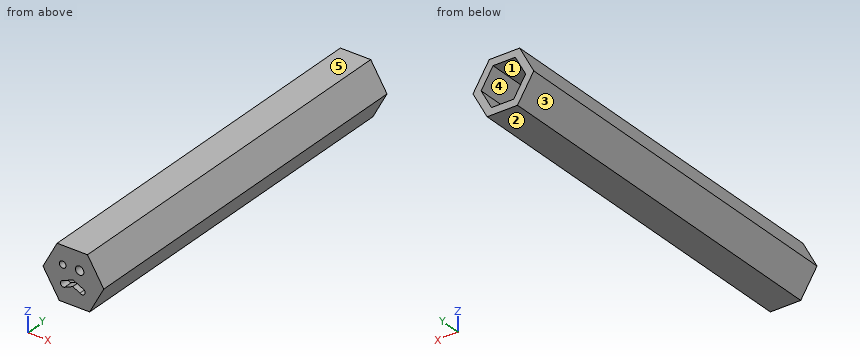
from build123d import *

# Parameters (mm, degrees)
F1_DEPTH = 31.75
F2_R     = 0.5886867957
F2_R_2   = 0.7557919615
F3_DEPTH = 1.5875


with BuildPart() as f1:
    # F0 (on Front) → F1 (new body, symmetric)
    with BuildSketch(Plane.XZ):
        Polygon((5.4726746476, 0.2241786608), (2.5421929086, 4.8515646018), (-2.930481739, 4.6273859411), (-5.4726746476, -0.2241786608), (-2.5421929086, -4.8515646018), (2.930481739, -4.6273859411), align=None)
        Polygon((-2.1458815411, 3.3884606556), (1.8615522369, 3.5526182559), (4.0074337781, 0.1641576003), (2.1458815411, -3.3884606556), (-1.8615522369, -3.5526182559), (-4.0074337781, -0.1641576003), align=None, mode=Mode.SUBTRACT)
    extrude(amount=F1_DEPTH, both=True)

    # F2 (on face) → F3 (join)
    with BuildSketch(Plane.XZ.offset(31.75)):
        Polygon((-2.5421929086, -4.8515646018), (2.930481739, -4.6273859411), (5.4726746476, 0.2241786608), (2.5421929086, 4.8515646018), (-2.930481739, 4.6273859411), (-5.4726746476, -0.2241786608), align=None)
        Polygon((-1.8615522369, -3.5526182559), (-4.0074337781, -0.1641576003), (-2.1458815411, 3.3884606556), (1.8615522369, 3.5526182559), (4.0074337781, 0.1641576003), (2.1458815411, -3.3884606556), align=None, mode=Mode.SUBTRACT)
        Polygon((-2.1458815411, 3.3884606556), (-4.0074337781, -0.1641576003), (-1.8615522369, -3.5526182559), (2.1458815411, -3.3884606556), (4.0074337781, 0.1641576003), (1.8615522369, 3.5526182559), align=None)
        with BuildLine():
            ThreePointArc((-1.6080282877, -2.2762045416), (-2.3121206431, -1.9400866098), (-1.90285574, -1.2758400079))
            Line((-1.90285574, -1.2758400079), (-0.0846300536, -0.4070492287))
            Line((-0.0846300536, -0.4070492287), (1.6315181704, -1.1626920101))
            ThreePointArc((1.6315181704, -1.1626920101), (1.7606026884, -1.201756272), (1.8765772228, -1.270594755))
            ThreePointArc((1.8765772228, -1.270594755), (1.9710769764, -2.063707268), (1.1761976946, -2.1419670217))
            Line((1.1761976946, -2.1419670217), (-0.1107579301, -1.5566768125))
            Line((-0.1107579301, -1.5566768125), (-1.5564763423, -2.2514307564))
            ThreePointArc((-1.5564763423, -2.2514307564), (-1.5819143346, -2.2645209548), (-1.6080282877, -2.2762045416))
        make_face(mode=Mode.SUBTRACT)
        with Locations((-1.9266997697, 1.430987264)):
            Circle(F2_R, mode=Mode.SUBTRACT)
        with Locations((1.1305541266, 1.6205844004)):
            Circle(F2_R_2, mode=Mode.SUBTRACT)
    extrude(amount=F3_DEPTH)


solid = f1.part
Could you check a few things on this model? Use its own coordinates, in mm. Face numbers are marked on the shaded views. A direction names the side the tool comes from. Give positions to 0.01 mm unless a question says otherwise; leave off trailing zeros. Order: outer loops, then holes, each group sorted by start corner. A loop starts at its lowest first (then second) coordinate and runs counter-clockwise, first axis right, second up.
1. Suppose I cut it at A-A (y = -17.5). Write out the boundary of the cut face in (x, z), plus the area to 3 significant figures.
Answers below:
outline: (-5.47, -0.22) - (-2.54, -4.85) - (2.93, -4.63) - (5.47, 0.22) - (2.54, 4.85) - (-2.93, 4.63) - close; hole (-4.01, -0.16) - (-1.86, -3.55) - (2.15, -3.39) - (4.01, 0.16) - (1.86, 3.55) - (-2.15, 3.39) - close
area: 36.1 mm2
2. I need wall thicknesses on L1, parallel to Y at x = -0.75, z = 0.75; L2, parallel to Z at x = -3.75, y = -24; L3, parallel to X at y = -6, z = -1. Which ranges of each line are inside material? Lowest first, please.
Answers below:
L1: y = -33.34 to -31.75
L2: z = -2.94 to -0.57, 0.33 to 3.06
L3: x = -4.98 to -3.48, 3.4 to 4.83
3. Which directions (+Z, -Z, +X, -X, +Y, -Y) give clear straight access to the entire face, cutting with the end or side of a thin tool? Please do the marked faces 1 and 2.
Answers below:
face 1: +Y
face 2: -Z, +X, +Y, -Y
4. For pin 1 (1.4 mm diameter, centred on x = 1.13, z = 1.62, fed in from +Y); pin 2 (1 mm diameter, centred on x = 4, y = -13.5, fed in from -Z); pin 3 (4 mm diameter, centred on x = -2.5, y = -3.5, fed in from +Z); pin 4 (1.5 mm diameter, centred on x = -1.93, z = 1.43, fed in from -Y), each with a flat end and sliding along its axis, tell me the tip position at first contact or that it passes through.
Answers below:
pin 1: passes through
pin 2: stops at z = -3.54
pin 3: stops at z = 4.73
pin 4: stops at y = -33.34
5. Thinking about a two-plate mould opening in Z: for the marked faces 3, 4 and 5, which applies, +Z half, -Z half, draft (parallel to the pull), parting line (faces both ways), or undercut?
Answers below:
face 3: -Z half
face 4: undercut
face 5: +Z half
